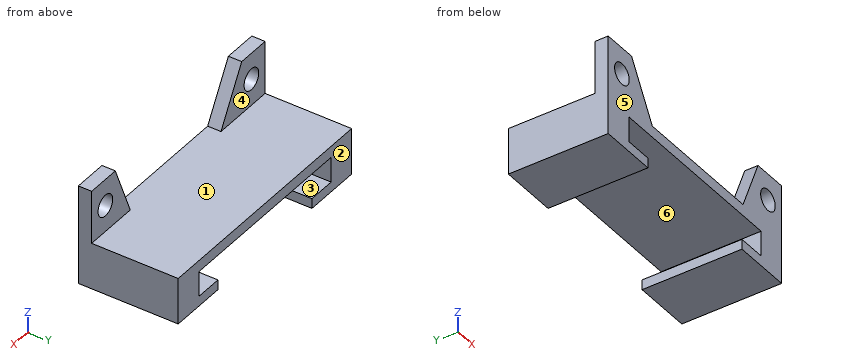
from build123d import *

# Parameters (mm, degrees)
F0_W      = 38
F0_H      = 15
F1_DEPTH  = 7
F2_W      = 29
F2_H      = 3.8
F3_DEPTH  = 30
F5_W      = 20.6003077328
F5_H      = 15
F6_DEPTH  = 5
F4_W      = 38
F4_H      = 2
F7_DEPTH  = 8
F9_D      = 3.2
F10_DEPTH = 25


with BuildPart() as f1:
    # F0 (on Top) → F1 (new body)
    with BuildSketch(Plane.XY):
        Rectangle(F0_W, F0_H)
    extrude(amount=F1_DEPTH)

    # F2 (on face) → F3 (cut)
    with BuildSketch(Plane.XZ.offset(7.5)):
        with Locations((0, 3.4002120374)):
            Rectangle(F2_W, F2_H)
    extrude(amount=-F3_DEPTH, mode=Mode.SUBTRACT)

    # F5 (on face) → F6 (cut)
    with BuildSketch(Plane(origin=(0, 0, 0), x_dir=(1, 0, 0), z_dir=(0, 0, -1))):
        Rectangle(F5_W, F5_H)
    extrude(amount=-F6_DEPTH, mode=Mode.SUBTRACT)

    # F4 (on face) → F7 (join)
    with BuildSketch(Plane.XY.offset(7)):
        with Locations((0, -6.5)):
            Rectangle(F4_W, F4_H)
    extrude(amount=F7_DEPTH)

    # F9 (through all)
    with Locations(Plane(origin=(0, -5.5, 0), x_dir=(-1, 0, 0), z_dir=(0, 1, 0))):
        with Locations((16, 11), (-16, 11)):
            Hole(F9_D / 2)

    # F8 (on face) → F10 (cut)
    with BuildSketch(Plane(origin=(0, -5.5, 0), x_dir=(-1, 0, 0), z_dir=(0, 1, 0))):
        Polygon((9.3329623342, 7), (13.877848681, 15), (-13.8199780472, 15), (-10.5432244018, 7), align=None)
    extrude(amount=-F10_DEPTH, mode=Mode.SUBTRACT)


solid = f1.part
The listing builds one solid part. Answer for the finished solid, in the listing's coordinates (mm). Face numbers are marked on the shaded views. A direction names the side the tool comes from. Coordinates: 2 decimals unless noted, no trailing zeros. Write each loop counter-clockwise with the first axis right and the second up, starting at its lowest first coordinate (ties: lowest second). Pieces come first, ordered by that corner, then holes. Notation, with made-up numbers: (-24.5, 30.25) - (-6.5, 30.25) arc R16 ccw to (-6.5, 48.25) - close; hole circle Ø10 at (2.5, 63.5). An arc over 180 degrees is marked (long way). Return JSON: item names as keys, results as strings.
1. The part is cut by section B-B on z = 2.5. Determine the outline of the cut face in (x, y), then the cut area to 3 significant figures.
Final values:
{"outline": "(-19, -7.5) - (-14.5, -7.5) - (-14.5, 7.5) - (-19, 7.5) - close; (14.5, -7.5) - (19, -7.5) - (19, 7.5) - (14.5, 7.5) - close", "area": "135 mm^2"}
2. The part is cut by section D-D on y = -3.25. Determine the outline of the cut face in (x, z), then the cut area to 3 significant figures.
Final values:
{"outline": "(-19, 0) - (-10.3, 0) - (-10.3, 1.5) - (-14.5, 1.5) - (-14.5, 5.3) - (14.5, 5.3) - (14.5, 1.5) - (10.3, 1.5) - (10.3, 0) - (19, 0) - (19, 7) - (-19, 7) - close", "area": "125 mm^2"}
3. The part is cut by section C-C on z = 12.25. Determine the outline of the cut face in (x, y).
Final values:
{"outline": "(-19, -7.5) - (-17, -7.5) - (-17, -5.5) - (-19, -5.5) - close; (-15, -7.5) - (-12.32, -7.5) - (-12.32, -5.5) - (-15, -5.5) - close; (12.69, -7.5) - (15, -7.5) - (15, -5.5) - (12.69, -5.5) - close; (17, -7.5) - (19, -7.5) - (19, -5.5) - (17, -5.5) - close"}
4. Consider line 1 along Z through (x, y) = (-16, -6.6); line 2 along X through (y, z) = (3.25, 0.75); line 3 along X through (y, z) = (2, 3.25). Determine where each line is inside the solid, lowest interval first.
Final values:
{"line 1": "0 to 9.4, 12.6 to 15", "line 2": "-19 to -10.3, 10.3 to 19", "line 3": "-19 to -14.5, 14.5 to 19"}
5. Each of these flat-tipped pins is pushed along its axis until it touches: pin 1 Ø3.5 at (x, z) = (16, 11) entering from -Y; pin 2 Ø1.5 at (x, y) = (3, 3.5) entering from +Z; pin 3 Ø2.5 at (x, z) = (-16, 11) entering from +Y; pin 4 Ø2.5 at (x, z) = (13.5, 10) entering from +Y. Where does it stop, or does it pass through?
Final values:
{"pin 1": "y = -7.5", "pin 2": "z = 7", "pin 3": "through", "pin 4": "y = -5.5"}
6. Which of the six approach directions +Z, -Z, +X, -X, +Y, -Y give full straight-line access (tool end or side, diameter ignored) to the marked faces 4, 5 and 6?
Final values:
{"face 4": "+Z, +X, -X, +Y", "face 5": "+Z, -Z, +X, -X, -Y", "face 6": "+Y, -Y"}
7. For a pull along Z with two mould halves and no side action, classify the marked faces 1, 2 and 3 as +Z half, -Z half, draft (parallel to the pull), parting line (faces both ways), or undercut.
Final values:
{"face 1": "+Z half", "face 2": "draft", "face 3": "undercut"}
8. The part is cut by section A-A on x = -16. Determine the outline of the cut face in (y, z), then the cut area to 3 significant figures.
Final values:
{"outline": "(-7.5, 0) - (7.5, 0) - (7.5, 7) - (-5.5, 7) - (-5.5, 9.4) - (-7.5, 9.4) - close; (-7.5, 12.6) - (-5.5, 12.6) - (-5.5, 15) - (-7.5, 15) - close", "area": "115 mm^2"}
